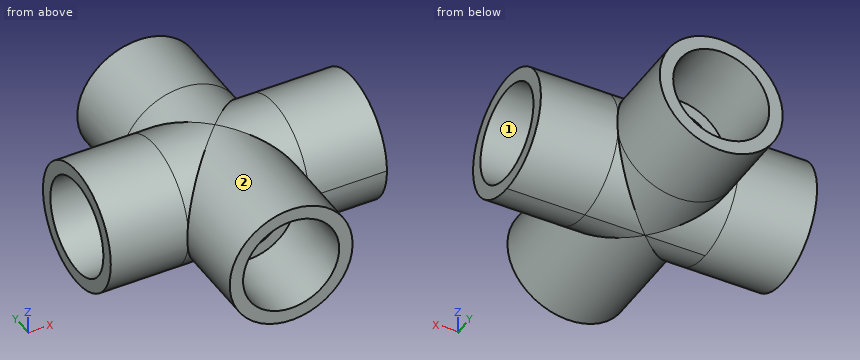
from build123d import *

# Parameters (mm, degrees)
SKETCH4_R           = 13.7795
BOSS_EXTRUDE1_DEPTH = 44.45
SKETCH5_R           = 13.7795
BOSS_EXTRUDE2_DEPTH = 44.45


with BuildPart() as part:
    # Sketch1 → Revolve1 (revolve)
    with BuildSketch(Plane.XY):
        Polygon((-30.95625, -13.7795), (-13.49375, -13.7795), (-13.49375, -10.6172), (-30.95625, -10.7696), align=None)
        Polygon((30.95625, -10.7696), (13.49375, -10.6172), (13.49375, -13.7795), (30.95625, -13.7795), align=None)
    revolve(axis=Axis((-30.95625, 0, 0), (1, 0, 0)))



with BuildPart() as body_2:
    # Sketch2 → Revolve2 (revolve)
    with BuildSketch(Plane.XY):
        Polygon((10.7696, 30.95625), (10.6172, 13.49375), (13.7795, 13.49375), (13.7795, 30.95625), align=None)
        Polygon((13.7795, -30.95625), (10.7696, -30.95625), (10.6172, -13.49375), (13.7795, -13.49375), align=None)
    revolve(axis=Axis((0, 0, 0), (0, 1, 0)))


with BuildPart() as part_1:
    add(part.part)

    add(body_2.part)  # Boss-Extrude1 merges body 2
    # Sketch4 → Boss-Extrude1 (add)
    with BuildSketch(Plane(origin=(-13.49375, 0, 0), x_dir=(0, 0, -1), z_dir=(1, 0, 0))):
        Circle(SKETCH4_R)
    extrude(amount=BOSS_EXTRUDE1_DEPTH)

    # Sketch5 → Boss-Extrude2 (add)
    with BuildSketch(Plane.XZ.offset(-13.49375)):
        Circle(SKETCH5_R)
    extrude(amount=BOSS_EXTRUDE2_DEPTH)

    # Sketch6 → Cut-Revolve1 (revolve, cut)
    with BuildSketch(Plane.XY):
        Polygon((-30.95625, -10.7696), (-13.49375, -10.6172), (-13.49375, -7.8994), (13.49375, -7.8994), (13.49375, -10.6172), (30.95625, -10.7696), (30.95625, 0), (-30.95625, 0), align=None)
    revolve(axis=Axis((30.95625, 0, 0), (-1, 0, 0)), mode=Mode.SUBTRACT)

    # Sketch7 → Cut-Revolve2 (revolve, cut)
    with BuildSketch(Plane.XY):
        Polygon((10.7696, 30.95625), (10.6172, 13.49375), (7.8994, 13.49375), (7.8994, -13.49375), (10.6172, -13.49375), (10.7696, -30.95625), (0, -30.95625), (0, 30.95625), align=None)
    revolve(axis=Axis((0, 30.95625, 0), (0, -1, 0)), mode=Mode.SUBTRACT)


solid = part_1.part
Can you work these out from the model? Positions are in its coordinate system, mm. Face numbers are marked on the shaded views. Coordinates: 2 decimals unless noted, no trailing zeros. Write each loop counter-clockwise with the first axis right and the second up, starting at its lowest first coordinate (ties: lowest second). Pieces come first, ordered by that corner, then holes.
Q1. Imagine slicing it at A-A, the plane y = -16. List the corners of the cut face in (x, z) for me, plus the area to 3 significant figures.
Results found:
outline: circle Ø27.56 at (0, 0); hole circle Ø21.28 at (0, 0)
area: 241 mm2
Q2. Please list where these lines run through material, in increasing order: L1, parallel to Z at x = 14, y = 0; L2, parallel to Z at x = 0, y = -4.25; L3, parallel to Y at x = 8.5, z = 0.
Results found:
L1: z = -13.78 to -10.62, 10.62 to 13.78
L2: z = -13.78 to -7.9, 7.9 to 13.78
L3: y = -13.49 to -7.9, 7.9 to 13.49
Q3. If we mould it in two halves opening along Z, with no side actions, what happens to the marked faces 1 and 2? For each: +Z half, -Z half, draft (parallel to the pull), parting line (faces both ways), or undercut.
Results found:
face 1: undercut
face 2: parting line
Q4. Imagine slicing it at B-B, the plane z = 4.25. Count the separate pieces of the cut face and the enclosed holes in it, plus the area to 3 significant figures.
Results found:
separate pieces: 4
enclosed holes: 0
area: 647 mm2
Q5. For P1, Ø1.5, axis at x = -11, y = 11.5, coming from the -Z side; P2, Ø1.5, axis at y = -17, z = -10.5, coming from the -X side; P3, Ø4, axis at x = -4.5, z = -8, coming from the +Y side; P4, Ø14, axis at x = 0, z = 0, coming from the +Y side, each with a flat end and sliding along its axis, tell me the tip position at first contact or that it passes through.
Results found:
P1: stops at z = -9.21
P2: stops at x = -9.74
P3: stops at y = 30.96
P4: passes through
Q6. Imagine slicing it at C-C, the plane x = 18.5. List the corners of the cut face in (y, z) for me.
Results found:
outline: circle Ø27.56 at (0, 0); hole circle Ø21.32 at (0, 0)
